Source: CAD feature listing. Evaluate the final solid. Frame: model axes, mm. Face numbers are marked on the shaded views. Round coordinates to 2 decimals unless told otherwise and drop trailing zeros. Order: outer loops, then holes, each group sorted by start corner. A loop starts at its lowest first (then second) coordinate and runs counter-clockwise, first axis right, second up. Notation, with made-up numbers: (8.5, 59.5) - (25.5, 59.5) arc R7 cw to (25.5, 71.5) - close; hole circle Ø4 at (25.25, 38.25). An arc over 180 degrees is marked (long way). Put each result on its own line as item: value. Start each with the question number.
1) Section B-B on x = 59.5. Output: boundary loops of the cut face in (y, z).
2) Section A-A on y = 0. Output: boundary loops of the cut face in (x, z), then the cut area to 3 significant figures.
3) Mould query, pull axis X, two halves, no side actions, for the marked faces 1 and 2. Classes: +X half, -X half, draft (parallel to the pull), parting line (faces both ways), or undercut.
4) Line query: probe 1 along Y at (x, z) = (46.5, 2.75); probe 2 along Y at (x, z) = (26.5, 1.5); probe 3 along X at (y, z) = (-1, 1). Output: solid intervals per line, ascending. Write a range as [from, to].
5) Section C-C on y = 4. Output: boundary loops of the cut face in (x, z), then the cut area to 3 significant figures.
6) Contact query for flat-ended pins moving along their axis: P1, Ø1, axis at y = 10.5, z = 3, coming from the +X side; P2, Ø2, axis at x = 37, z = 4, coming from the +Y side; P3, Ø2, axis at y = -3, z = 4, coming from the +X side. Output: stop coordinate, or through.
```python
from build123d import *

# Parameters (mm, degrees)
SKETCH2_R           = 2.65
BOSS_EXTRUDE2_DEPTH = 6


with BuildPart() as part:
    # Sketch2 → Boss-Extrude2 (new body)
    with BuildSketch(Plane.XY):
        with BuildLine():
            add(Edge.make_bspline(
                [(45, 16.035396523), (44.644632939, 15.999223801), (41.619048326, 15.685620583), (36.155474951, 15.030554758), (29.005619164, 13.923317691), (24.539912926, 13.049943774), (22.5, 12.599580353)],
                knots=[0.418410632, 0.418410632, 0.418410632, 0.418410632, 0.420162443, 0.433328265, 0.445393603, 0.455638041, 0.455638041, 0.455638041, 0.455638041], degree=3))
            ThreePointArc((22.5, 12.599580353), (38.184673742, 0), (22.5, -12.599580353))
            add(Edge.make_bspline(
                [(22.5, -12.599580353), (24.539912926, -13.049943774), (29.005619164, -13.923317691), (36.155474951, -15.030554758), (41.619048326, -15.685620583), (44.644632939, -15.999223801), (45, -16.035396523)],
                knots=[0.544361959, 0.544361959, 0.544361959, 0.544361959, 0.554606397, 0.566671735, 0.579837557, 0.581589368, 0.581589368, 0.581589368, 0.581589368], degree=3))
            ThreePointArc((45, -16.035396523), (62.750493933, 0), (45, 16.035396523))
        make_face()
        with Locations((46.632238895, 0)):
            Circle(SKETCH2_R, mode=Mode.SUBTRACT)
    extrude(amount=BOSS_EXTRUDE2_DEPTH)


solid = part.part
```
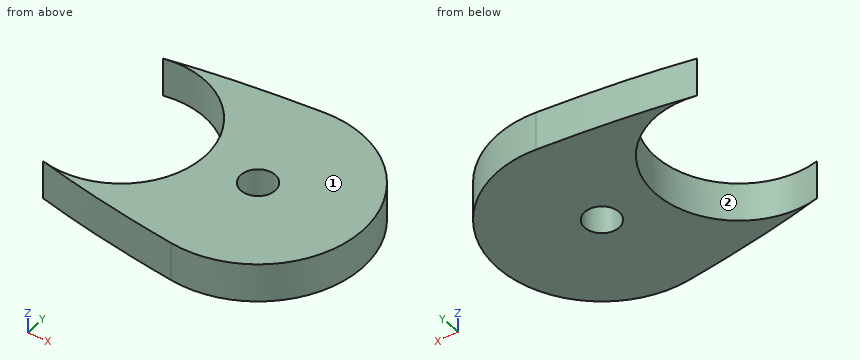
Answer sheet:
1. outline: (-9.71, 0) - (9.71, 0) - (9.71, 6) - (-9.71, 6) - close
2. outline: (38.18, 0) - (43.98, 0) - (43.98, 6) - (38.18, 6) - close; (49.28, 0) - (62.75, 0) - (62.75, 6) - (49.28, 6) - close
2. area: 116 mm^2
3. face 1: draft
3. face 2: undercut
4. probe 1: [-16.12, -2.65], [2.65, 16.12]
4. probe 2: [-13.42, -12.85], [12.85, 13.42]
4. probe 3: [38.15, 44.18], [49.09, 62.72]
5. outline: (37.55, 0) - (62.25, 0) - (62.25, 6) - (37.55, 6) - close
5. area: 148 mm^2
6. P1: x = 59.27
6. P2: y = 15.23
6. P3: x = 62.63
